Here's how the part is built. I have some questions about the finished solid (model axes, mm). Give positions to 0.01 mm unless a question says otherwise; leave off trailing zeros. Write each loop counter-clockwise with the first axis right and the second up, starting at its lowest first coordinate (ties: lowest second). Pieces come first, ordered by that corner, then holes. Notation, with made-up numbers: (61, 48.5) - (107, 48.5) arc R15 ccw to (107, 60.5) - close; hole circle Ø11 at (-29, -18). An arc over 180 degrees is marked (long way). Use a Markdown table: item, result.
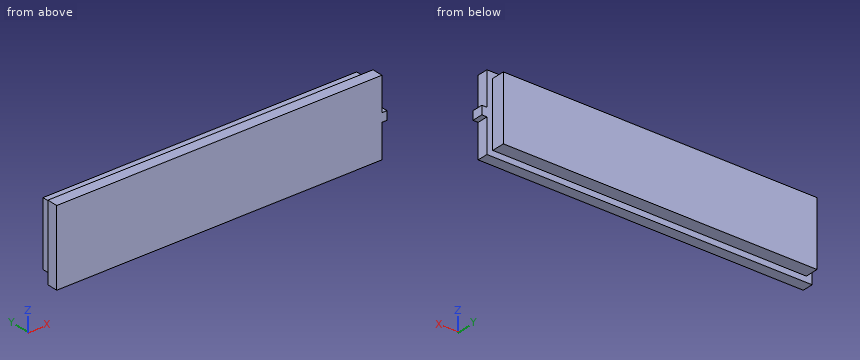
```python
from build123d import *

# Parameters (mm, degrees)
BOSS_EXTRUDE1_DEPTH = 1.9
SKETCH2_W           = 54.62
SKETCH2_H           = 11.24
BOSS_EXTRUDE2_DEPTH = 2.3


with BuildPart() as part:
    # Sketch1 → Boss-Extrude1 (new body)
    with BuildSketch(Plane(origin=(0, 0, 0), x_dir=(1, 0, 0), z_dir=(0, 1, 0))):
        Polygon((28.31, 6.615), (28.31, 0.75), (29.21, 0.75), (29.21, -0.75), (28.31, -0.75), (28.31, -6.615), (-28.31, -6.615), (-28.31, 6.615), align=None)
    extrude(amount=BOSS_EXTRUDE1_DEPTH)

    # Sketch2 → Boss-Extrude2 (add)
    with BuildSketch(Plane(origin=(0, 1.9, 0), x_dir=(1, 0, 0), z_dir=(0, 1, 0))):
        Rectangle(SKETCH2_W, SKETCH2_H)
    extrude(amount=BOSS_EXTRUDE2_DEPTH)


solid = part.part
```
Item 1: If we section it at A-A, the plane z = -3.75: Write out the boundary of the cut face in (x, y), plus the area to 3 significant figures.
Values:
| item | result |
|---|---|
| outline | (-28.31, 0) - (28.31, 0) - (28.31, 1.9) - (27.31, 1.9) - (27.31, 4.2) - (-27.31, 4.2) - (-27.31, 1.9) - (-28.31, 1.9) - close |
| area | 233 mm2 |
Item 2: Will these pins go through, and if not, where does the flat tip stop? pin 1 Ø2 at (y, z) = (1.5, -2.5) entering from +X; pin 2 Ø1.1 at (x, y) = (-7, 3) entering from -Z; pin 3 Ø1.8 at (x, y) = (13.5, 3.5) entering from +Z.
Values:
| item | result |
|---|---|
| pin 1 | stops at x = 28.31 |
| pin 2 | stops at z = -5.62 |
| pin 3 | stops at z = 5.62 |
Item 3: If we section it at B-B, the plane x = 12: Write out the boundary of the cut face in (y, z) (3 decimals), plus the area to 3 significant figures.
Values:
| item | result |
|---|---|
| outline | (0, -6.615) - (1.9, -6.615) - (1.9, -5.62) - (4.2, -5.62) - (4.2, 5.62) - (1.9, 5.62) - (1.9, 6.615) - (0, 6.615) - close |
| area | 51.0 mm2 |
Item 4: I need wall thicknesses on line 1 along X through (y, z) = (0.95, 3.75); line 2 along Z through (x, y) = (5, 2); line 3 along X through (y, z) = (2.6, -1.5). Which ranges of each line are inside material? Lowest first, please. Write a range as [from, to].
Values:
| item | result |
|---|---|
| line 1 | x = [-28.31, 28.31] |
| line 2 | z = [-5.62, 5.62] |
| line 3 | x = [-27.31, 27.31] |
Item 5: If we section it at C-C, the plane y = 3.2: Write out the boundary of the cut face in (x, z).
Values:
| item | result |
|---|---|
| outline | (-27.31, -5.62) - (27.31, -5.62) - (27.31, 5.62) - (-27.31, 5.62) - close |
